Geometry: see drawing. Coordinates: mm, zero at the bounding-box minimum. Give positions to 0.01 mm unless a question says otherwise; leave off trailing zeros. Loops run counter-clockwise (first coordinate to the right, second up) from the corner with the lowest first, then second, coordinate; pieces in that order, holes last. Notation, with made-up numbers: (87, -3) -> (105, -3) arc R17 cw to (105, 25) -> close; hole circle Ø4 at (28.5, -7.75). An arc over 180 degrees is marked (long way). Answer in a Markdown table with one row per item. Add a question column.
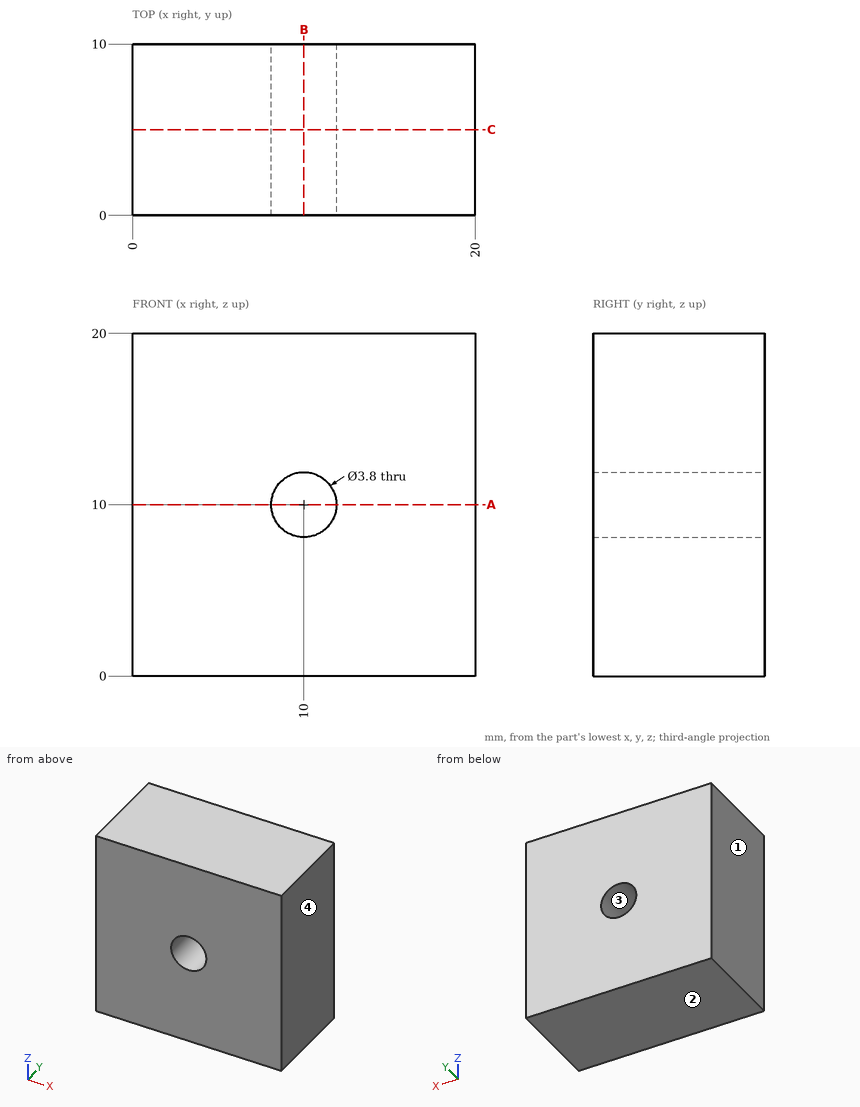
1) Material intervals for line 1 along Z through (x, y) = (10, 7.5); line 2 along Z through (x, y) = (9, 9.75), sorted ascending.
2) Section B-B on x = 10. Output: boundary loops of the cut face in (y, z).
3) Pull-direction query (X, two-part tool) for the marked faces 1, 2, 3 and 4; classes: +X half, -X half, draft (parallel to the pull), parting line (faces both ways), or undercut.
4) Section A-A on z = 10. Output: boundary loops of the cut face in (x, y), and give its area (3 significant figures).
5) Section C-C on y = 5. Output: boundary loops of the cut face in (x, z).
Working result:
| question | item | result |
|---|---|---|
| 1 | line 1 | z = 0 to 8.1, 11.9 to 20 |
| 1 | line 2 | z = 0 to 8.38, 11.62 to 20 |
| 2 | outline | (0, 0) -> (10, 0) -> (10, 8.1) -> (0, 8.1) -> close; (0, 11.9) -> (10, 11.9) -> (10, 20) -> (0, 20) -> close |
| 3 | face 1 | -X half |
| 3 | face 2 | draft |
| 3 | face 3 | undercut |
| 3 | face 4 | +X half |
| 4 | outline | (0, 0) -> (8.1, 0) -> (8.1, 10) -> (0, 10) -> close; (11.9, 0) -> (20, 0) -> (20, 10) -> (11.9, 10) -> close |
| 4 | area | 162 mm2 |
| 5 | outline | (0, 0) -> (20, 0) -> (20, 20) -> (0, 20) -> close; hole circle Ø3.8 at (10, 10) |
